Autodesk Inventor part; units mm, degrees
ref_plane "YZ Plane" through (0, 0, 0) normal (1, 0, 0) x (0, 1, 0)
ref_plane "XZ Plane" through (0, 0, 0) normal (0, 1, 0) x (-1, 0, 0)
ref_plane "XY Plane" through (0, 0, 0) normal (0, 0, 1) x (1, 0, 0)
sketch "Sketch1" plane through (0, 0, 0) normal (0, 1, 0) x (-1, 0, 0)
  line L0 (-5, 6) -> (5, 6)
  line L1 (5, 6) -> (5, -6)
  line L2 (5, -6) -> (-5, -6)
  line L3 (-5, -6) -> (-5, 6)
  line L4 (-5, 6) -> (5, -6) construction
  line L5 (5, 6) -> (-5, -6) construction
  circle A0 centre (0, 0) radius 1.5
  line L6 (5, 0) -> (-5, 0) construction
  line L7 (0, 6) -> (0, -6) construction
  circle A1 centre (0, 4.5) radius 0.8
  circle A2 centre (0, -4.5) radius 0.8
  dimension "d0" = 10
  dimension "d1" = 12
  dimension "d2" = 3
  dimension "d3" = 9
  dimension "d4" = 1.6
extrude "Extrusion1" add sketch "Sketch1" along normal blind 0.8
fillet "Fillet1" radius 0.5 4 edges at (-5, 0.4, 6) (5, 0.4, 6) (5, 0.4, -6) (-5, 0.4, -6)
sketch "Sketch2" plane through (0, 0.8, 0) normal (0, 1, 0) x (1, 0, 0)
  circle A0 centre (0, 0) radius 1.5
  circle A1 centre (0, 0) radius 2
  dimension "d9" = 4
extrude "Extrusion2" add sketch "Sketch2" along normal blind 0.8
properties part number "Encoder Front Plate" material "Brass, Soft Yellow"
For this review, take the finished solid that the model builds, in its own axes (mm). Round coordinates to 2 decimals unless told otherwise and drop trailing zeros. Write each loop counter-clockwise with the first axis right and the second up, starting at its lowest first coordinate (ties: lowest second). Pieces come first, ordered by that corner, then holes. Notation, with made-up numbers: M 63,87 L 89,87 A16 ccw 89,95 Z; hole C 81,40 d11. An arc over 180 degrees is marked long. Write item = value, one per line. Start each with the question number.
(1) We need section C-C (y = 0.25). Give the boundary of the cut face in (x, z), then the cut area to 3 significant figures.
(2) We need section A-A (z = -4.5). Give the boundary of the cut face in (x, y), then the cut area to 3 significant figures.
(3) For line 1 along Z through (x, y) = (0, 0.35); line 2 along X through (y, z) = (0.3, 0); line 3 along Z through (x, y) = (0, 1.2), list the stretches that pass through material, from the lowest coordinate up.
(4) Clearance check with a flat-ended pin moving along its axis: pin 1 Ø2.5 at (x, z) = (0, 4.5) entering from +Y. State where the tip first meets the part, or that it passes through.
(5) We need section B-B (x = 0). Give the boundary of the cut face in (y, z), then the cut area to 3 significant figures.
(6) The part is to be moulded in two halves that separate along X. For faces 1 (the face through (0, 1, -2)), 2 (the face through (0.17, 0.39, -3.72)), 3 (the face through (1.2, 0, 1.4)), say which applies: +X half, -X half, draft (parallel to the pull), parting line (faces both ways), or undercut.
(7) We need section D-D (z = 0). Give the boundary of the cut face in (x, y), then the cut area to 3 significant figures.
Results found:
q1.outline = M -5,-5.5 A0.5 ccw -4.5,-6 L 4.5,-6 A0.5 ccw 5,-5.5 L 5,5.5 A0.5 ccw 4.5,6 L -4.5,6 A0.5 ccw -5,5.5 Z; hole C 0,0 d3; hole C 0,-4.5 d1.6; hole C 0,4.5 d1.6
q1.area = 109 mm²
q2.outline = M -5,0 L -0.8,0 L -0.8,0.8 L -5,0.8 Z; M 0.8,0 L 5,0 L 5,0.8 L 0.8,0.8 Z
q2.area = 6.72 mm²
q3.line_1 = -6 to -5.3, -3.7 to -1.5, 1.5 to 3.7, 5.3 to 6
q3.line_2 = -5 to -1.5, 1.5 to 5
q3.line_3 = -2 to -1.5, 1.5 to 2
q4.pin_1 = 0.8
q5.outline = M 0,-6 L 0.8,-6 L 0.8,-5.3 L 0,-5.3 Z; M 0,-3.7 L 0.8,-3.7 L 0.8,-2 L 1.6,-2 L 1.6,-1.5 L 0,-1.5 Z; M 0,1.5 L 1.6,1.5 L 1.6,2 L 0.8,2 L 0.8,3.7 L 0,3.7 Z; M 0,5.3 L 0.8,5.3 L 0.8,6 L 0,6 Z
q5.area = 5.44 mm²
q6.face_1 = parting line
q6.face_2 = undercut
q6.face_3 = draft
q7.outline = M -5,0 L -1.5,0 L -1.5,1.6 L -2,1.6 L -2,0.8 L -5,0.8 Z; M 1.5,0 L 5,0 L 5,0.8 L 2,0.8 L 2,1.6 L 1.5,1.6 Z
q7.area = 6.40 mm²
